Could you check a few things on this model? Use its own coordinates, in mm. A direction names the side the tool comes from. Give positions to 0.01 mm unless a question says otherwise; leave off trailing zeros. Write each loop counter-clockwise with the first axis right and the second up, starting at its lowest first coordinate (ties: lowest second). Pieces come first, ordered by that corner, then holes. Notation, with made-up numbers: (48.25, -30) -> (72.25, -30) arc R13 cw to (72.25, -12) -> close; hole circle Ø5 at (10, -16). An arc over 180 degrees is marked (long way). Write item = value, one per line. Start each with the question number.
```python
from build123d import *

# Parameters (mm, degrees)
SALIENTE_EXTRUIR1_DEPTH = 177.8
CROQUIS2_W              = 177.8
CROQUIS2_H              = 558.8
CORTAR_EXTRUIR1_DEPTH   = 25.4
VACIADO1_START          = -323.85
VACIADO1_DEPTH          = 647.7
VACIADO1_2_OUTLINE_W    = 6.35
VACIADO1_2_OUTLINE_H    = 215.9
VACIADO1_2_DEPTH        = 88.9


# Read off the part's stored shape, not the designer's step: Vaciado1
with BuildPart() as part:
    # Croquis1 → Saliente-Extruir1 (new, symmetric)
    with BuildSketch(Plane.XY):
        Polygon((-133.35, 342.9), (-133.35, -342.9), (133.35, -342.9), (133.35, 0), (133.35, 342.9), align=None)
    extrude(amount=SALIENTE_EXTRUIR1_DEPTH, both=True)

    # Croquis2 → Cortar-Extruir1 (cut)
    with BuildSketch(Plane(origin=(133.35, 0, 0), x_dir=(0, 0, -1), z_dir=(1, 0, 0))):
        with Locations((0, 63.5)):
            Rectangle(CROQUIS2_W, CROQUIS2_H)
    extrude(amount=-CORTAR_EXTRUIR1_DEPTH, mode=Mode.SUBTRACT)

    # Vaciado1 outline → Vaciado1 (cut)
    with BuildSketch(Plane(origin=(0, 0, 0), x_dir=(1, 0, 0), z_dir=(0, 1, 0)).offset(VACIADO1_START)):
        Polygon((-114.3, 158.75), (-114.3, -158.75), (114.3, -158.75), (114.3, -107.95), (107.95, -107.95), (107.95, 107.95), (114.3, 107.95), (114.3, 158.75), align=None)
    extrude(amount=VACIADO1_DEPTH, mode=Mode.SUBTRACT)

    # Vaciado1 2 outline → Vaciado1 2 (cut)
    with BuildSketch(Plane(origin=(0, 0, 0), x_dir=(1, 0, 0), z_dir=(0, 1, 0)).offset(VACIADO1_START)):
        with Locations((111.125, 0)):
            Rectangle(VACIADO1_2_OUTLINE_W, VACIADO1_2_OUTLINE_H)
    extrude(amount=VACIADO1_2_DEPTH, mode=Mode.SUBTRACT)


solid = part.part
```
(1) On a 3-axis mill with a long thin cutter (end or side, diameter ignored), from which of +Z, -Z, +X, -X, +Y, -Y can I reach the whole of each face in a straight line? I mean faces 1 (the flat face through (107.95, 334, 1)), 2 (the flat face through (-133.35, 5, 2)), 3 (the flat face through (2, -5, -158.75)). Say none if no direction works.
(2) Imagine slicing it at B-B (y = 60). Please give me the cut outline in (x, z), then the cut area to 3 significant figures.
(3) If I drill on line 1 along Z through (x, y) = (92, -297); line 2 along Y through (x, z) = (-98, -81.5); line 3 along X through (y, z) = (-217, -142), over which ranges is the centre line in solid material (lowest first)? Write a range as from..to.
(4) We'd pull the mould along Z, two halves only. Please class faces 4 (the flat face through (-2, 5, 177.8)), 5 (the flat face through (133.35, -81, 121)), 6 (the flat face through (-2, -5, 158.75)), 7 (the flat face through (-2, 5, -177.8)): released by +Z, released by -Z, zero draft, split by the parting line, or undercut.
(5) Imagine slicing it at A-A (x = -28.5). Please give me the cut outline in (y, z).
(6) Imagine slicing it at D-D (z = 36.5). Please give me the cut outline in (x, y), then the cut area to 3 significant figures.
(7) Imagine slicing it at C-C (z = 118.5). Please give me the cut outline in (x, y), then the cut area to 3 significant figures.
(8) I'm going to push flat-ended pins straight in: pin 1 (21 mm diameter, centred on y = 337.5, z = 21, fed in from +X); pin 2 (7.5 mm diameter, centred on x = 114.5, z = -12.5, fed in from +Y). Where does each tip first touch, or does it pass through?
Answers below:
q1.face_1 = +X, +Y
q1.face_2 = +Z, -Z, -X, +Y, -Y
q1.face_3 = none
q2.outline = (-133.35, -177.8) -> (133.35, -177.8) -> (133.35, -88.9) -> (107.95, -88.9) -> (107.95, -107.95) -> (114.3, -107.95) -> (114.3, -158.75) -> (-114.3, -158.75) -> (-114.3, 158.75) -> (114.3, 158.75) -> (114.3, 107.95) -> (107.95, 107.95) -> (107.95, 88.9) -> (133.35, 88.9) -> (133.35, 177.8) -> (-133.35, 177.8) -> close
q2.area = 19,100 mm^2
q3.line_1 = -177.8..-158.75, 158.75..177.8
q3.line_2 = -342.9..-323.85, 323.85..342.9
q3.line_3 = -133.35..-114.3, 114.3..133.35
q4.face_4 = released by +Z
q4.face_5 = zero draft
q4.face_6 = undercut
q4.face_7 = released by -Z
q5.outline = (-342.9, -177.8) -> (342.9, -177.8) -> (342.9, 177.8) -> (-342.9, 177.8) -> close; hole (-323.85, -158.75) -> (323.85, -158.75) -> (323.85, 158.75) -> (-323.85, 158.75) -> close
q6.outline = (-133.35, -342.9) -> (133.35, -342.9) -> (133.35, -215.9) -> (107.95, -215.9) -> (107.95, -234.95) -> (114.3, -234.95) -> (114.3, -323.85) -> (-114.3, -323.85) -> (-114.3, 323.85) -> (107.95, 323.85) -> (107.95, 342.9) -> (-133.35, 342.9) -> close
q6.area = 24,200 mm^2
q7.outline = (-133.35, -342.9) -> (133.35, -342.9) -> (133.35, 342.9) -> (-133.35, 342.9) -> close; hole (-114.3, -323.85) -> (114.3, -323.85) -> (114.3, 323.85) -> (-114.3, 323.85) -> close
q7.area = 34,800 mm^2
q8.pin_1 = 107.95
q8.pin_2 = -215.9
